Geometry: final body of the model. Coordinates: model frame, mm. Give positions to 0.01 mm unless a question says otherwise; leave off trailing zeros. Write each loop counter-clockwise with the first axis right and the second up, starting at its lowest first coordinate (ties: lowest second). Pieces come first, ordered by that corner, then holes.
Q1. Line query: line 1 (X direction, y = -70.5, z = -18); line 2 (Z direction, x = 56.5, y = -68.5); line 3 (X direction, y = -67.5, z = 63.5). Output: solid intervals per line, ascending.
Q2. Section B-B (x = 0). Return the cut outline in (y, z), plus the area to 3 significant figures.
Q3. Section A-A (z = 0). Return the cut outline in (x, y), plus the area to 3 significant figures.
Q4. Section D-D (x = -72). Return the cut outline in (y, z).
Q5. Pin query (flat end, axial travel): pin 1 Ø1.5 at (y, z) = (-72, 9.5) entering from +X; pin 2 Ø1 at (y, z) = (-69, 8.5) entering from +X. Return the tip coordinate at first contact, or that it passes through.
Q6. Section C-C (y = -70.25). State how many separate pieces and enclosed holes the cut face has, plus the area to 3 significant figures.
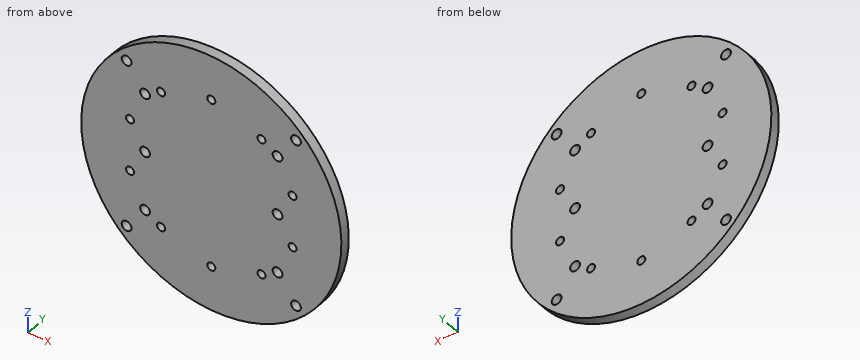
from build123d import *

# Parameters (mm, degrees)
SKETCH1_R           = 84.1675
SKETCH1_R_2         = 3.175
SKETCH1_R_3         = 2.6035
BOSS_EXTRUDE1_DEPTH = 6.35


with BuildPart() as part:
    # Sketch1 → Boss-Extrude1 (new body)
    with BuildSketch(Plane.XZ.offset(66.8)):
        with Locations(Location((0, 0, 0), (0, 0, 270))):
            Circle(SKETCH1_R)
        with Locations(Location((54.800775542, 54.800775542, 0), (0, 0, 270))):
            Circle(SKETCH1_R_2, mode=Mode.SUBTRACT)
        with Locations(Location((54.800775542, -54.800775542, 0), (0, 0, 270))):
            Circle(SKETCH1_R_2, mode=Mode.SUBTRACT)
        with Locations(Location((-54.800775542, -54.800775542, 0), (0, 0, 270))):
            Circle(SKETCH1_R_2, mode=Mode.SUBTRACT)
        with Locations(Location((-54.800775542, 54.800775542, 0), (0, 0, 270))):
            Circle(SKETCH1_R_2, mode=Mode.SUBTRACT)
        with Locations(Location((-42.8625, -38.476238101, 0), (0, 0, 270))):
            Circle(SKETCH1_R_2, mode=Mode.SUBTRACT)
        with Locations(Location((-42.8625, 0, 0), (0, 0, 270))):
            Circle(SKETCH1_R_2, mode=Mode.SUBTRACT)
        with Locations(Location((-42.8625, 38.476238101, 0), (0, 0, 270))):
            Circle(SKETCH1_R_2, mode=Mode.SUBTRACT)
        with Locations(Location((42.8625, 38.476238101, 0), (0, 0, 270))):
            Circle(SKETCH1_R_2, mode=Mode.SUBTRACT)
        with Locations(Location((42.8625, 0, 0), (0, 0, 270))):
            Circle(SKETCH1_R_2, mode=Mode.SUBTRACT)
        with Locations(Location((42.8625, -38.476238101, 0), (0, 0, 270))):
            Circle(SKETCH1_R_2, mode=Mode.SUBTRACT)
        with Locations(Location((-52.598201949, -17.0901918, 0), (0, 0, 270))):
            Circle(SKETCH1_R_3, mode=Mode.SUBTRACT)
        with Locations(Location((-52.598201949, 17.0901918, 0), (0, 0, 270))):
            Circle(SKETCH1_R_3, mode=Mode.SUBTRACT)
        with Locations(Location((-32.507476552, 44.742703006, 0), (0, 0, 270))):
            Circle(SKETCH1_R_3, mode=Mode.SUBTRACT)
        with Locations(Location((0, 55.305022413, 0), (0, 0, 270))):
            Circle(SKETCH1_R_3, mode=Mode.SUBTRACT)
        with Locations(Location((32.507476552, 44.742703006, 0), (0, 0, 270))):
            Circle(SKETCH1_R_3, mode=Mode.SUBTRACT)
        with Locations(Location((52.598201949, 17.0901918, 0), (0, 0, 270))):
            Circle(SKETCH1_R_3, mode=Mode.SUBTRACT)
        with Locations(Location((52.598201949, -17.0901918, 0), (0, 0, 270))):
            Circle(SKETCH1_R_3, mode=Mode.SUBTRACT)
        with Locations(Location((32.507476552, -44.742703006, 0), (0, 0, 270))):
            Circle(SKETCH1_R_3, mode=Mode.SUBTRACT)
        with Locations(Location((0, -55.305022413, 0), (0, 0, 270))):
            Circle(SKETCH1_R_3, mode=Mode.SUBTRACT)
        with Locations(Location((-32.507476552, -44.742703006, 0), (0, 0, 270))):
            Circle(SKETCH1_R_3, mode=Mode.SUBTRACT)
    extrude(amount=BOSS_EXTRUDE1_DEPTH)


solid = part.part
Computed:
1. line 1: x = -82.22 to -55.04, -50.16 to 50.16, 55.04 to 82.22
1. line 2: z = -62.39 to -57.48, -52.12 to 52.12, 57.48 to 62.39
1. line 3: x = -55.24 to 55.24
2. outline: (-73.15, -84.17) - (-66.8, -84.17) - (-66.8, -57.91) - (-73.15, -57.91) - close; (-73.15, -52.7) - (-66.8, -52.7) - (-66.8, 52.7) - (-73.15, 52.7) - close; (-73.15, 57.91) - (-66.8, 57.91) - (-66.8, 84.17) - (-73.15, 84.17) - close
2. area: 1,000 mm2
3. outline: (-84.17, -73.15) - (-46.04, -73.15) - (-46.04, -66.8) - (-84.17, -66.8) - close; (-39.69, -73.15) - (39.69, -73.15) - (39.69, -66.8) - (-39.69, -66.8) - close; (46.04, -73.15) - (84.17, -73.15) - (84.17, -66.8) - (46.04, -66.8) - close
3. area: 988 mm2
4. outline: (-73.15, -43.59) - (-66.8, -43.59) - (-66.8, 43.59) - (-73.15, 43.59) - close
5. pin 1: stops at x = 83.71
5. pin 2: stops at x = 83.79
6. separate pieces: 1
6. enclosed holes: 20
6. area: 21,700 mm2
